Print and shaded views of the part. All mm, measured from the part's lowest x, y and z. Round coordinates to 2 decimals unless told otherwise and drop trailing zeros. Write each loop counter-clockwise with the first axis right and the second up, starting at its lowest first coordinate (ties: lowest second). Pieces come first, ordered by that corner, then holes.
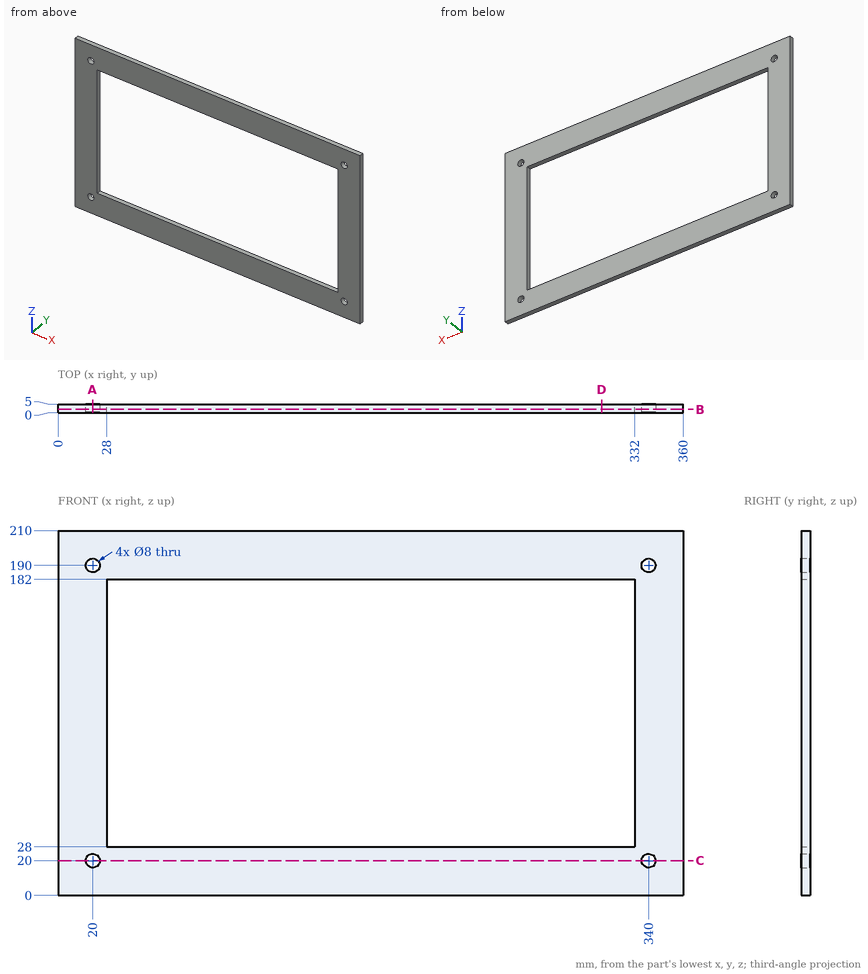
1) Slice it at B-B (y = 1.85). Write the cut outline in (x, z), plus the area to 3 significant figures.
Results:
outline: (0, 0) - (360, 0) - (360, 210) - (0, 210) - close; hole circle Ø8 at (20, 20); hole circle Ø8 at (20, 190); hole (28, 28) - (332, 28) - (332, 182) - (28, 182) - close; hole circle Ø8 at (340, 20); hole circle Ø8 at (340, 190)
area: 28,600 mm2
2) Slice it at A-A (x = 20). Write the cut outline in (y, z).
Results:
outline: (0, 0) - (5, 0) - (5, 16) - (0, 16) - close; (0, 24) - (5, 24) - (5, 186) - (0, 186) - close; (0, 194) - (5, 194) - (5, 210) - (0, 210) - close
3) Wall check: L1, parallel to Z at x = 20, y = 1.35; L2, parallel to X at y = 1.45, z = 20; L3, parallel to X at y = 2.75, z = 122.5. Give the ranges that are in metal, low to high.
Results:
L1: z = 0 to 16, 24 to 186, 194 to 210
L2: x = 0 to 16, 24 to 336, 344 to 360
L3: x = 0 to 28, 332 to 360
4) Slice it at D-D (x = 313). Write the cut outline in (y, z), plus the area to 3 significant figures.
Results:
outline: (0, 0) - (5, 0) - (5, 28) - (0, 28) - close; (0, 182) - (5, 182) - (5, 210) - (0, 210) - close
area: 280 mm2
5) Slice it at C-C (z = 20). Write the cut outline in (x, y).
Results:
outline: (0, 0) - (16, 0) - (16, 5) - (0, 5) - close; (24, 0) - (336, 0) - (336, 5) - (24, 5) - close; (344, 0) - (360, 0) - (360, 5) - (344, 5) - close
